Build history of the part. All positions in model axes, mm. A direction names the side the tool comes from. Round coordinates to 2 decimals unless told otherwise and drop trailing zeros. Write each loop counter-clockwise with the first axis right and the second up, starting at its lowest first coordinate (ties: lowest second). Pieces come first, ordered by that corner, then holes.
from build123d import *

# Parameters (mm, degrees)
SKETCH2_R                = 8
SKETCH2_R_2              = 7
BOSS_EXTRUDE3_DEPTH      = 15
BOSS_EXTRUDE6_DEPTH      = 11
BOSS_EXTRUDE6_DEPTH_BACK = 40
SKETCH4_R                = 8
SKETCH4_R_2              = 7
SKETCH3_R                = 9
SKETCH3_R_2              = 8
BOSS_EXTRUDE7_DEPTH      = 60
SKETCH6_R                = 8
SKETCH6_R_2              = 7
BOSS_EXTRUDE8_DEPTH      = 31


with BuildPart() as part:
    # Sketch2 → Boss-Extrude3 (new body)
    with BuildSketch(Plane(origin=(0, 0, 0), x_dir=(1, 0, 0), z_dir=(0, 1, 0))):
        with Locations(Location((0, 0, 0), (0, 0, 270))):
            Circle(SKETCH2_R)
        with Locations(Location((0, 0, 0), (0, 0, 270))):
            Circle(SKETCH2_R_2, mode=Mode.SUBTRACT)
    extrude(amount=BOSS_EXTRUDE3_DEPTH)

    # Sketch4 → Boss-Extrude6 (add, two sides: drawn at the far end of the back side and taken through both)
    with BuildSketch(Plane(origin=(0, 45, 0), x_dir=(1, 0, 0), z_dir=(0, 1, 0)).offset(-BOSS_EXTRUDE6_DEPTH_BACK)):
        with Locations(Location((0, 0, 0), (0, 0, 270))):
            Circle(SKETCH4_R)
        with Locations(Location((0, 0, 0), (0, 0, 270))):
            Circle(SKETCH4_R_2, mode=Mode.SUBTRACT)
    extrude(amount=BOSS_EXTRUDE6_DEPTH + BOSS_EXTRUDE6_DEPTH_BACK)

    # Sketch3 → Boss-Extrude7 (add)
    with BuildSketch(Plane(origin=(0, 10, 0), x_dir=(1, 0, 0), z_dir=(0, 1, 0))):
        with Locations(Location((0, 0, 0), (0, 0, 90))):
            Circle(SKETCH3_R)
        with Locations(Location((0, 0, 0), (0, 0, 270))):
            Circle(SKETCH3_R_2, mode=Mode.SUBTRACT)
    extrude(amount=BOSS_EXTRUDE7_DEPTH)

    # Sketch6 → Boss-Extrude8 (add)
    with BuildSketch(Plane(origin=(0, 45, 0), x_dir=(1, 0, 0), z_dir=(0, 1, 0))):
        with Locations(Location((0, 0, 0), (0, 0, 270))):
            Circle(SKETCH6_R)
        with Locations(Location((0, 0, 0), (0, 0, 270))):
            Circle(SKETCH6_R_2, mode=Mode.SUBTRACT)
    extrude(amount=BOSS_EXTRUDE8_DEPTH)


solid = part.part
1) Mould opens along X. For faces 4 (the flat face through (-6, 76, 4)), 5 (the cylindrical face through (-6.834, 37.468, -1.517)), 6 (the cylindrical face through (-2.703, 39.58, -8.584)) say: released by +X, released by -X, zero draft, split by the parting line, or undercut.
Results:
face 4: zero draft
face 5: undercut
face 6: split by the parting line
2) Which spindle directions (+Z, -Z, +X, -X, +Y, -Y) get a long thin tool onto all of the face, cutting with end or side? Do faces 1 (the cylindrical face through (-7.81, 72.96, -1.73)), 2 (the cylindrical face through (-7.81, 4.93, -1.73)), 3 (the flat face through (-6, 0, 4)). Say none if no direction does.
Results:
face 1: +Y
face 2: -Y
face 3: +Z, -Z, +X, -X, -Y
3) Slice it at C-C (y = 32). Write the cut outline in (x, z), plus the area to 3 significant figures.
Results:
outline: circle Ø18 at (0, 0); hole circle Ø14 at (0, 0)
area: 101 mm2
4) Slice it at A-A (x = 0). Write the cut outline in (y, z), plus the area to 3 significant figures.
Results:
outline: (0, -8) - (10, -8) - (10, -9) - (70, -9) - (70, -8) - (76, -8) - (76, -7) - (0, -7) - close; (0, 7) - (76, 7) - (76, 8) - (70, 8) - (70, 9) - (10, 9) - (10, 8) - (0, 8) - close
area: 272 mm2
5) Pin check, flat tips, straight feed: pin 1 Ø4 at (x, z) = (-3, 3.5) entering from +Y; pin 2 Ø5.5 at (x, z) = (3, 4) entering from -Y; pin 3 Ø1.5 at (y, z) = (23, 2) entering from -X; pin 4 Ø4 at (x, y) = (6.5, 34) entering from +Z. Stop position of each tip, or through.
Results:
pin 1: passes through
pin 2: stops at y = 0
pin 3: stops at x = -8.91
pin 4: stops at z = 7.79
6) Wall check: L1, parallel to X at y = 18, z = 0; L2, parallel to Y at x = -7, z = 4.75; L3, parallel to X at y = 63, z = 5. Give the ranges that are in metal, low to high.
Results:
L1: x = -9 to -7, 7 to 9
L2: y = 10 to 70
L3: x = -7.48 to -4.9, 4.9 to 7.48
7) Slice it at B-B (z = 0). Write the cut outline in (x, y).
Results:
outline: (-9, 10) - (-8, 10) - (-8, 0) - (-7, 0) - (-7, 76) - (-8, 76) - (-8, 70) - (-9, 70) - close; (7, 0) - (8, 0) - (8, 10) - (9, 10) - (9, 70) - (8, 70) - (8, 76) - (7, 76) - close
